Part print with two shaded views. Sizes in mm from the minimum x, y, z corner. A direction names the side the tool comes from. Give positions to 0.01 mm unless a question says otherwise; leave off trailing zeros. Write each loop counter-clockwise with the first axis right and the second up, starting at its lowest first coordinate (ties: lowest second). Pieces come first, ordered by that corner, then holes. Notation, with made-up numbers: (25.5, 13) - (63.5, 13) arc R16 cw to (63.5, 18) - close; hole circle Ø11 at (61.5, 27.5). An arc over 180 degrees is marked (long way). One line per item, written item: value. Start each with the question number.
(1) 3-axis set-ups, long thin cutter, end or side, ignore diameter. For the marked faces 1, 2 and 3: which of +Z, -Z, +X, -X, +Y, -Y reach the whole face in a straight line?
(2) Cut at C-C, the plane y = 12.75. List the corners of the cut face in (x, z), and give its area (3 significant figures).
(3) Probe L1, parallel to Y at x = 8.5, z = 1; L2, parallel to Y at x = 11, z = 9; L3, parallel to Z at x = 9, y = 7.75. List the from-to ranges inside material, lowest first.
(4) Cut at A-A, the plane x = 8. List the corners of the cut face in (y, z).
(5) Cut at B-B, the plane z = 8. List the corners of the cut face in (x, y).
(6) Cut at D-D, the plane x = 4.5. List the corners of the cut face in (y, z).
(7) Drop flat-ended pins along their axis: P1, Ø4, axis at y = 5.5, z = 10.5, coming from the -X side; P2, Ø2, axis at x = 13, z = 11, coming from the +Y side; P3, Ø8, axis at y = 4.5, z = 8.5, coming from the +X side; P4, Ø2, axis at x = 10, y = 5.5, coming from the +Z side. Give the stop position or say it passes through.
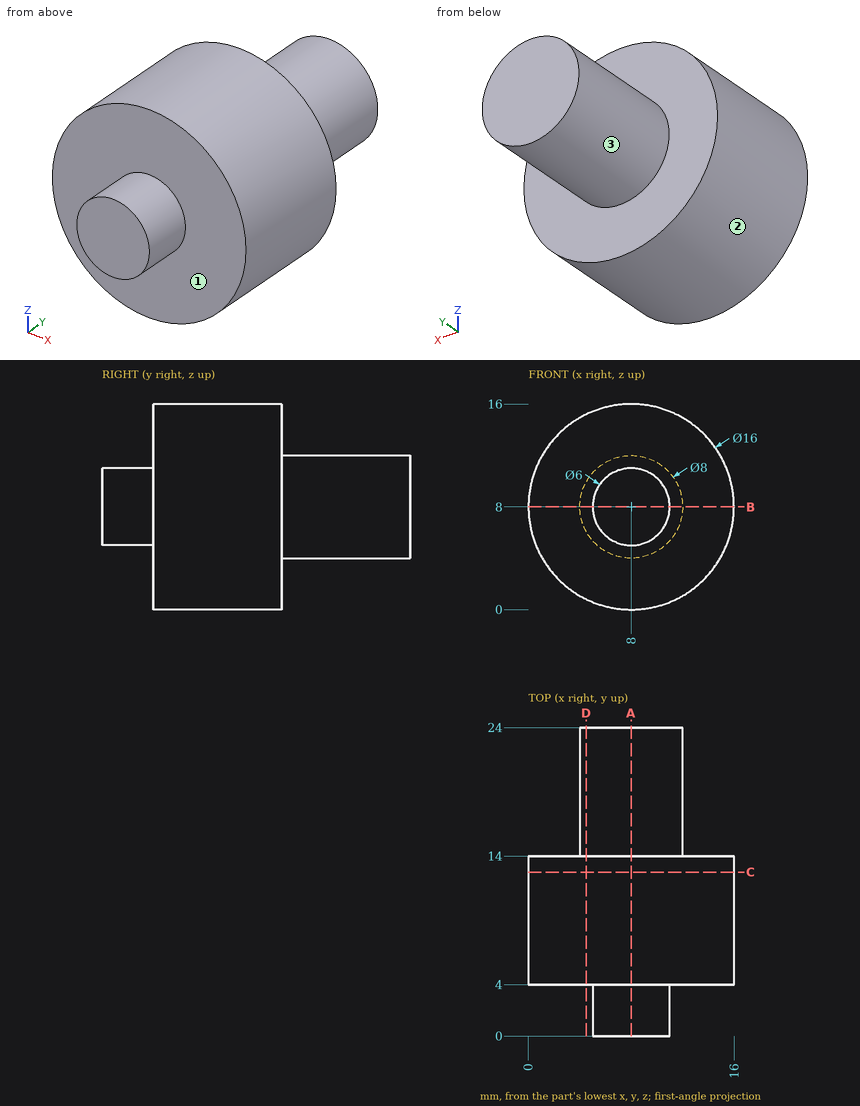
Answers follow:
1. face 1: -Y
1. face 2: +Y, -Y
1. face 3: +Y
2. outline: circle Ø16 at (8, 8)
2. area: 201 mm²
3. L1: y = 4 to 14
3. L2: y = 4 to 24
3. L3: z = 0.06 to 15.94
4. outline: (0, 5) - (4, 5) - (4, 0) - (14, 0) - (14, 4) - (24, 4) - (24, 12) - (14, 12) - (14, 16) - (4, 16) - (4, 11) - (0, 11) - close
5. outline: (0, 4) - (5, 4) - (5, 0) - (11, 0) - (11, 4) - (16, 4) - (16, 14) - (12, 14) - (12, 24) - (4, 24) - (4, 14) - (0, 14) - close
6. outline: (4, 0.81) - (14, 0.81) - (14, 6.06) - (24, 6.06) - (24, 9.94) - (14, 9.94) - (14, 15.19) - (4, 15.19) - close
7. P1: stops at x = 0.02
7. P2: stops at y = 14
7. P3: stops at x = 16
7. P4: stops at z = 15.94
